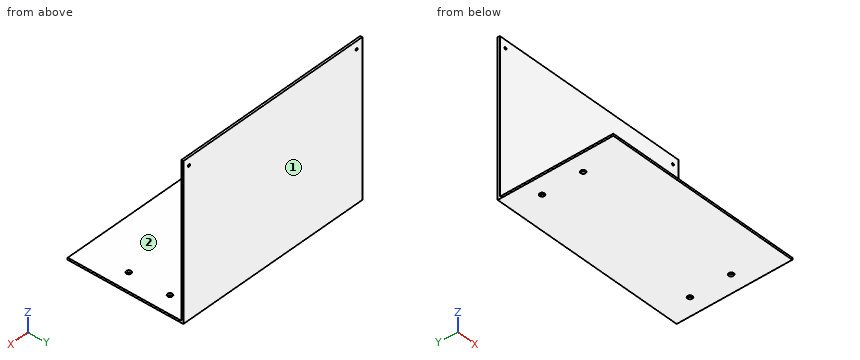
from build123d import *

# Parameters (mm, degrees)
SKETCH1_W               = 291.5
SKETCH1_H               = 168.5
BOSS_EXTRUDE1_DEPTH     = 3
F_1_4_CLEARANCE_HOLE1_D = 7.14248
SKETCH6_W               = 291.5
SKETCH6_H               = 3
BOSS_EXTRUDE2_DEPTH     = 222.5
TAP_DRILL_FOR_M4_TAP2_D = 3.3


with BuildPart() as part:
    # Sketch1 → Boss-Extrude1 (new body)
    with BuildSketch(Plane.XY):
        with Locations((145.75, -84.25)):
            Rectangle(SKETCH1_W, SKETCH1_H)
    extrude(amount=BOSS_EXTRUDE1_DEPTH)

    # 1/4 Clearance Hole1 (through all)
    with Locations(Plane.XY.offset(3)):
        with Locations((25.25, -102), (25.25, -42), (266.25, -42), (266.25, -102)):
            Hole(F_1_4_CLEARANCE_HOLE1_D / 2)

    # Sketch6 → Boss-Extrude2 (add)
    with BuildSketch(Plane.XY.offset(3)):
        with Locations((145.75, -1.5)):
            Rectangle(SKETCH6_W, SKETCH6_H)
    extrude(amount=BOSS_EXTRUDE2_DEPTH)

    # Tap Drill for M4 Tap2 (through all)
    with Locations(Plane(origin=(0, 0, 0), x_dir=(1, 0, 0), z_dir=(0, 1, 0))):
        with Locations((9.25, -214), (282.25, -214)):
            Hole(TAP_DRILL_FOR_M4_TAP2_D / 2)


solid = part.part
Geometry check sheet. Reference: the model listing, model coordinates, mm. Face numbers are marked on the shaded views. A direction names the side the tool comes from. Give positions to 0.01 mm unless a question says otherwise; leave off trailing zeros. Order: outer loops, then holes, each group sorted by start corner. A loop starts at its lowest first (then second) coordinate and runs counter-clockwise, first axis right, second up.
1. Sectioned sample at A-A (x = 266.25). Record the boundary of the cut face in (y, z), then the cut area to 3 significant figures.
Completed:
outline: (-168.5, 0) - (-105.57, 0) - (-105.57, 3) - (-168.5, 3) - close; (-98.43, 0) - (-45.57, 0) - (-45.57, 3) - (-98.43, 3) - close; (-38.43, 0) - (0, 0) - (0, 225.5) - (-3, 225.5) - (-3, 3) - (-38.43, 3) - close
area: 1,130 mm2
2. Depth check by flat-ended pin: pin 1 (4.5 mm diameter, centred on x = 266.25, y = -102, fed in from -Z); pin 2 (11.5 mm diameter, centred on x = 25.25, y = -42, fed in from +Z). Enter the tip coordinate at first touch or a pass-through.
Completed:
pin 1: passes through
pin 2: stops at z = 3
3. Sectioned sample at C-C (x = 91). Record the boundary of the cut face in (y, z), then the cut area to 3 significant figures.
Completed:
outline: (-168.5, 0) - (0, 0) - (0, 225.5) - (-3, 225.5) - (-3, 3) - (-168.5, 3) - close
area: 1,170 mm2
4. Sectioned sample at D-D (y = -31.5). Record the boundary of the cut face in (x, z).
Completed:
outline: (0, 0) - (291.5, 0) - (291.5, 3) - (0, 3) - close
5. Scan lines: line 1 (Y direction, x = 266.25, z = 0.7); line 2 (X direction, y = -0.95, z = 214); line 3 (Z direction, x = 9.25, y = -1.95). Record each from-to range of solid material in increasing order.
Completed:
line 1: y = -168.5 to -105.57, -98.43 to -45.57, -38.43 to 0
line 2: x = 0 to 7.6, 10.9 to 280.6, 283.9 to 291.5
line 3: z = 0 to 212.35, 215.65 to 225.5
6. Access from +Z, -Z, +X, -X, +Y, -Y to the whole of each face (thin tool, end or side, straight path). Record for the marked faces 1 and 2.
Completed:
face 1: +Z, -Z, +X, -X, +Y
face 2: +Z, +X, -X, -Y
7. Sectioned sample at B-B (y = -102). Record the boundary of the cut face in (x, z).
Completed:
outline: (0, 0) - (21.68, 0) - (21.68, 3) - (0, 3) - close; (28.82, 0) - (262.68, 0) - (262.68, 3) - (28.82, 3) - close; (269.82, 0) - (291.5, 0) - (291.5, 3) - (269.82, 3) - close
